Autodesk Inventor part; units mm, degrees
ref_plane "YZ Plane" through (0, 0, 0) normal (1, 0, 0) x (0, 1, 0)
ref_plane "XZ Plane" through (0, 0, 0) normal (0, 1, 0) x (-1, 0, 0)
ref_plane "XY Plane" through (0, 0, 0) normal (0, 0, 1) x (1, 0, 0)
sketch "Boceto1" plane through (0, 0, 0) normal (0, 1, 0) x (-1, 0, 0)
  line L0 (-20, -60) -> (20, -60)
  line L1 (20, -60) -> (20, 60)
  line L2 (20, 60) -> (-20, 60)
  line L3 (-20, 60) -> (-20, -60)
  line L4 (-20, -60) -> (20, 60) construction
  line L5 (20, -60) -> (-20, 60) construction
  line L6 (20, 60) -> (-20, 60)
  line L7 (-20, 60) -> (-20, 20)
  line L8 (-20, 20) -> (20, 20)
  line L9 (20, 20) -> (20, 60)
  line L10 (20, -60) -> (-20, -60)
  line L11 (-20, -60) -> (-20, -20)
  line L12 (-20, -20) -> (20, -20)
  line L13 (20, -20) -> (20, -60)
  circle A0 centre (0, 40) radius 10
  circle A1 centre (0, -40) radius 10
  line L14 (20, 20) -> (-20, 20)
  line L15 (-20, 20) -> (-20, -20)
  line L16 (-20, -20) -> (20, -20)
  line L17 (20, -20) -> (20, 20)
  point P0 (0, 0)
  dimension "d0" = 40
  dimension "d1" = 120
  dimension "d2" = 40
  dimension "d3" = 40
  dimension "d4" = 40
  dimension "d5" = 20
  dimension "d7" = 20
extrude "Extrusión1" add sketch "Boceto1" along normal blind 10
sketch "Boceto2" plane through (0, 10, 0) normal (0, 1, 0) x (1, 0, 0)
  line L0 (-20, -20) -> (20, -20)
  line L1 (20, -20) -> (20, 20)
  line L2 (20, 20) -> (-20, 20)
  line L3 (-20, 20) -> (-20, -20)
  line L4 (-20, -20) -> (20, 20) construction
  line L5 (20, -20) -> (-20, 20) construction
  point P0 (0, 0)
  dimension "d10" = 40
  dimension "d11" = 40
extrude "Extrusión2" add sketch "Boceto2" along normal blind 40
fillet "Empalme de cara1" radius 20 1 edges at (20, 5, 60)
fillet "Empalme de cara2" radius 20 1 edges at (-20, 5, 60)
fillet "Empalme de cara3" radius 20 1 edges at (-20, 5, -60)
fillet "Empalme de cara4" radius 20 1 edges at (20, 5, -60)
sketch "Boceto3" plane through (20, 10, -20) normal (1, 0, 0) x (0, 0, -1)
  line L0 (-60, 0) -> (-40, 0)
  circle A0 centre (-20, 20) radius 10
  point P0 (-20, -10)
  dimension "d22" = 20
extrude "Extrusión3" cut sketch "Boceto3" against normal blind 40
fillet "Empalme de cara5" radius 20 1 edges at (0, 50, 20)
fillet "Empalme de cara6" radius 20 1 edges at (0, 50, -20)
properties part number "Tarea 1"
Source: CAD feature listing. Evaluate the final solid. Frame: model axes, mm. A direction names the side the tool comes from. Round coordinates to 2 decimals unless told otherwise and drop trailing zeros. Loops run counter-clockwise (first coordinate to the right, second up) from the corner with the lowest first, then second, coordinate; pieces in that order, holes last. Notation, with made-up numbers: (39.25, 86) -> (73.25, 86) arc R5 ccw to (73.25, 91) -> close; hole circle Ø7 at (37, 67.25). An arc over 180 degrees is marked (long way). Answer as a JSON object with one key per item and string values. Group by question number.
Q1. Section query D-D (y = 34). Output: boundary loops of the cut face in (x, z), plus the area to 3 significant figures.
Q2. Access query for faces 5 (the cylindrical face through (13.986, 5.07, 54.297)), 6 (the flat face through (0, 10, 27)), 7 (the flat face through (0, 20, -20)). Directions: +Z, -Z, +X, -X, +Y, -Y. A direction counts if a zero-diameter tool reaches every point of the face in a straight line with its end or side. Return the directions, or none.
Q3. Contact query for flat-ended pins moving along their axis: P1, Ø10, axis at x = 14.5, y = 32.5, coming from the -Z side; P2, Ø5, axis at x = -13, y = 39.5, coming from the +Z side (3 decimals); P3, Ø4, axis at x = -6.5, y = 29, coming from the +Z side. Output: stop coordinate, or through.
Q4. Section query A-A (x = 4.5). State how many separate pieces and enclosed holes the cut face has, plus the area to 3 significant figures.
Q5. Ray query, line 1 (Z direction, x = 0, y = 7.25); line 2 (Y direction, x = 8, z = 0); line 3 (Y direction, x = -16.5, z = -43). Return the intervals inside material, ascending. Write a range as from..to.
Q6. Mould query, pull axis Z, two halves, no side actions, for faces 1 (the cylindrical face through (2.17, 4.93, 49.76)), 2 (the flat face through (-20, 19, -1)), 3 (the cylindrical face through (0.28, 20.24, 2.17)), 4 (the cylindrical face through (0.28, 44.297, 13.986)). Classes: pulls with the +Z half, pulls with the -Z half, needs draft (parallel to the pull), parting line crosses it, or undercut.
Completed:
{
 "1": {"outline": "(-20, -19.6) -> (20, -19.6) -> (20, -9.17) -> (-20, -9.17) -> close; (-20, 9.17) -> (20, 9.17) -> (20, 19.6) -> (-20, 19.6) -> close", "area": "834 mm²"},
 "2": {"face 5": "+Z, +X, +Y, -Y", "face 6": "+Z, +X, -X, +Y", "face 7": "-Z, +X, -X, +Y"},
 "3": {"P1": "z = -20", "P2": "z = 18.735", "P3": "z = 20"},
 "4": {"separate pieces": "3", "enclosed holes": "1", "area": "1,950 mm²"},
 "5": {"line 1": "-60..-50, -30..30, 50..60", "line 2": "0..20, 40..50", "line 3": "0..10"},
 "6": {"face 1": "undercut", "face 2": "needs draft", "face 3": "undercut", "face 4": "pulls with the +Z half"}
}
